Verification items for the finished model (mm, model axes). A direction names the side the tool comes from. Give positions to 0.01 mm unless a question says otherwise; leave off trailing zeros. Write each loop counter-clockwise with the first axis right and the second up, starting at its lowest first coordinate (ties: lowest second). Pieces come first, ordered by that corner, then holes. Notation, with made-up numbers: (30.5, 46.5) -> (87.5, 46.5) arc R23 cw to (87.5, 68.5) -> close; hole circle Ø9 at (14, 5.5). An arc over 180 degrees is marked (long way). Answer as CSV lines item,"result". Start each with the question number.
1) Sectioned sample at B-B on y = -2. Record the cut outline in (x, z).
2) Gauge pin test, flat ends, axial feed: pin 1 Ø1 at (y, z) = (-3, -1) entering from -X; pin 2 Ø1 at (y, z) = (-7.5, -4) entering from -X; pin 3 Ø10 at (y, z) = (10, 8) entering from -X. Record the tip position at first contact, or that the pin passes through.
3) Mould release check, pull along Y, two halves, no side actions. Record for faces 5 (the flat face through (-6, -19, -2)), 6 (the cylindrical face through (16.97, 11.62, -10.74)), 7 (the cylindrical face through (-5.57, -9.93, -5.38)): released by +Y, released by -Y, zero draft, split by the parting line, or undercut.
4) Material ranges on L1, parallel to X at y = -2.05, z = 0; L2, parallel to Y at x = 11, z = 0; L3, parallel to Z at x = -5, y = 15, recorded low to high.
5) Tool access check on faces 1 (the cylindrical face through (-24.74, -2.46, -2.38)), 2 (the flat face through (-4, -15, 2)), 3 (the flat face through (19, 12, -8)), 4 (the cylindrical face through (11.9, 16.4, -7.63)). Record the directions out of +Z, -Z, +X, -X, +Y, -Y that give a thin tool (end or side, any length) a straight path to the whole face; none if there is none.
6) Sectioned sample at A-A on x = 10.5. Record the cut outline in (y, z).
```python
from build123d import *

# Parameters (mm, degrees)
SWEEP_THIN1_PROFILE_R   = 11
SWEEP_THIN1_PROFILE_R_2 = 8
SKETCH70_R              = 10
SKETCH70_R_2            = 8
BOSS_EXTRUDE1_DEPTH     = 10
SKETCH71_R              = 11
SKETCH71_R_2            = 8
BOSS_EXTRUDE2_DEPTH     = 4
SKETCH72_R              = 10
SKETCH72_R_2            = 8
BOSS_EXTRUDE3_DEPTH     = 10
SKETCH73_R              = 11
SKETCH73_R_2            = 8
BOSS_EXTRUDE4_DEPTH     = 4


with BuildPart() as part:
    # Sweep-Thin1: sweep along a path in Sketch1
    with BuildLine(Plane.XY) as sweep_thin1_path:
        Line((-14, -5), (-14, 0))
        ThreePointArc((-14, 0), (-9.899495, 9.899495), (0, 14))
        Line((0, 14), (5, 14))
    # Sweep-Thin1 profile (on start of the path) → Sweep-Thin1 (sweep)
    with BuildSketch(Plane(origin=(-14, -5, 0), x_dir=(0, 0, 1), z_dir=(0, 1, 0))):
        Circle(SWEEP_THIN1_PROFILE_R)
        Circle(SWEEP_THIN1_PROFILE_R_2, mode=Mode.SUBTRACT)
    sweep(path=sweep_thin1_path.line)

    # Sketch70 → Boss-Extrude1 (add)
    with BuildSketch(Plane.XZ.offset(5)):
        with Locations(Location((-14, 0, 0), (0, 0, 270))):
            Circle(SKETCH70_R)
        with Locations(Location((-14, 0, 0), (0, 0, 180))):
            Circle(SKETCH70_R_2, mode=Mode.SUBTRACT)
    extrude(amount=BOSS_EXTRUDE1_DEPTH)

    # Sketch71 → Boss-Extrude2 (add)
    with BuildSketch(Plane.XZ.offset(15)):
        with Locations(Location((-14, 0, 0), (0, 0, 90))):
            Circle(SKETCH71_R)
        with Locations(Location((-14, 0, 0), (0, 0, 180))):
            Circle(SKETCH71_R_2, mode=Mode.SUBTRACT)
    extrude(amount=BOSS_EXTRUDE2_DEPTH)

    # Sketch72 → Boss-Extrude3 (add)
    with BuildSketch(Plane(origin=(5, 0, 0), x_dir=(0, 0, -1), z_dir=(1, 0, 0))):
        with Locations((0, 14)):
            Circle(SKETCH72_R)
        with Locations((0, 14)):
            Circle(SKETCH72_R_2, mode=Mode.SUBTRACT)
    extrude(amount=BOSS_EXTRUDE3_DEPTH)

    # Sketch73 → Boss-Extrude4 (add)
    with BuildSketch(Plane(origin=(15, 0, 0), x_dir=(0, 0, -1), z_dir=(1, 0, 0))):
        with Locations(Location((0, 14, 0), (0, 0, 90))):
            Circle(SKETCH73_R)
        with Locations((0, 14)):
            Circle(SKETCH73_R_2, mode=Mode.SUBTRACT)
    extrude(amount=BOSS_EXTRUDE4_DEPTH)


solid = part.part
```
Ans:
1,outline,"circle Ø22 at (-14, 0); hole circle Ø16 at (-14, 0)"
2,pin 1,"stops at x = -24.99"
2,pin 2,"stops at x = -23.37"
2,pin 3,"stops at x = -23.21"
3,face 5,"released by -Y"
3,face 6,"split by the parting line"
3,face 7,"undercut"
4,L1,"x = -25 to -22, -6 to -3"
4,L2,"y = 4 to 6, 22 to 24"
4,L3,"z = -10.85 to -7.79, 7.79 to 10.85"
5,face 1,"-Y"
5,face 2,"none"
5,face 3,"+Z, -Z, +X, +Y, -Y"
5,face 4,"+X"
6,outline,"circle Ø20 at (14, 0); hole circle Ø16 at (14, 0)"
